Source: CAD feature listing. Evaluate the final solid. Frame: model axes, mm. A direction names the side the tool comes from. Round coordinates to 2 decimals unless told otherwise and drop trailing zeros. Loops run counter-clockwise (first coordinate to the right, second up) from the corner with the lowest first, then second, coordinate; pieces in that order, holes last. Notation, with made-up numbers: M 44,44 L 67,44 A8 cw 67,57 Z; hole C 44.25,-7 d7. An arc over 180 degrees is marked long. One line per item, written item: value.
from build123d import *

# Parameters (mm, degrees)
SKETCH_1_R      = 4
SKETCH_1_R_2    = 1.5
EXTRUDE_1_DEPTH = 3.3
SKETCH_2_W      = 33
SKETCH_2_H      = 26.5
SKETCH_2_R      = 4.9
SKETCH_2_R_2    = 1.495427909
EXTRUDE_2_DEPTH = 3.3


with BuildPart() as part:
    # 草图1 → 凸台-拉伸1 (new body)
    with BuildSketch(Plane(origin=(0, 0, 0), x_dir=(0, 0, -1), z_dir=(1, 0, 0))):
        with BuildLine():
            Line((-13.25, 0), (-13.25, -20.75))
            Line((-13.25, -20.75), (13.25, -20.75))
            Line((13.25, -20.75), (13.25, 0))
            ThreePointArc((13.25, 0), (0, 13.25), (-13.25, 0))
        make_face()
        Circle(SKETCH_1_R, mode=Mode.SUBTRACT)
        with Locations((8.5, 0)):
            Circle(SKETCH_1_R_2, mode=Mode.SUBTRACT)
        with Locations(Location((-8.5, 0, 0), (0, 0, 180))):
            Circle(SKETCH_1_R_2, mode=Mode.SUBTRACT)
    extrude(amount=EXTRUDE_1_DEPTH)

    # 草图2 → 凸台-拉伸2 (add)
    with BuildSketch(Plane.XZ.offset(20.75)):
        with Locations((16.5, 0)):
            Rectangle(SKETCH_2_W, SKETCH_2_H)
        with Locations(Location((17.8, 0, 0), (0, 0, 270))):
            Circle(SKETCH_2_R, mode=Mode.SUBTRACT)
        with Locations(Location((24.85, -8, 0), (0, 0, 270))):
            Circle(SKETCH_2_R_2, mode=Mode.SUBTRACT)
        with Locations(Location((24.85, 8, 0), (0, 0, 90))):
            Circle(SKETCH_2_R_2, mode=Mode.SUBTRACT)
        with Locations(Location((10.75, 8, 0), (0, 0, 270))):
            Circle(SKETCH_2_R_2, mode=Mode.SUBTRACT)
        with Locations(Location((10.75, -8, 0), (0, 0, 90))):
            Circle(SKETCH_2_R_2, mode=Mode.SUBTRACT)
    extrude(amount=-EXTRUDE_2_DEPTH)


solid = part.part
1. Section query A-A (x = 24.85). Return the cut outline in (y, z), and give its area (3 significant figures).
Report:
outline: M -20.75,-13.25 L -17.45,-13.25 L -17.45,-9.5 L -20.75,-9.5 Z; M -20.75,-6.5 L -17.45,-6.5 L -17.45,6.5 L -20.75,6.5 Z; M -20.75,9.5 L -17.45,9.5 L -17.45,13.25 L -20.75,13.25 Z
area: 67.7 mm2
2. Reachability of faces 1 (the face through (3.3, -5, 0)), 2 (the face through (12.6, -20.75, 0.2)) from +Z, -Z, +X, -X, +Y, -Y: full face, straight path, thin tool, end or side. Return the list, or none.
Report:
face 1: +Z, -Z, +X, +Y
face 2: +Z, -Z, +X, -X, -Y
3. Pull-direction query (Z, two-part tool) for faces 3 (the face through (18, -17.45, 6)), 4 (the face through (10, -18, 13.25)), 5 (the face through (1.6, -0.9, -7.3)), 6 (the face through (1.627, 13.247, -0.291)); classes: released by +Z, released by -Z, zero draft, split by the parting line, or undercut.
Report:
face 3: zero draft
face 4: released by +Z
face 5: undercut
face 6: split by the parting line
4. Ray query, line 1 (X direction, y = -19, z = -8); line 2 (X direction, y = -18.5, z = 0); line 3 (X direction, y = -14, z = 2). Return the intervals inside material, ascending. Write a range as [from, to].
Report:
line 1: x = [0, 9.25], [12.25, 23.35], [26.35, 33]
line 2: x = [0, 12.9], [22.7, 33]
line 3: x = [0, 3.3]
5. Pin query (flat end, axial travel): pin 1 (2.5 mm diameter, centred on x = 24.85, z = -8, fed in from -Y); pin 2 (3 mm diameter, centred on x = 16.5, z = 3.5, fed in from -Y); pin 3 (4 mm diameter, centred on x = 29, z = 7, fed in from +Y); pin 4 (3.5 mm diameter, centred on y = 0, z = 8.5, fed in from +X). Return the tip coordinate at first contact, or that it passes through.
Report:
pin 1: passes through
pin 2: stops at y = -20.75
pin 3: stops at y = -17.45
pin 4: stops at x = 3.3
6. Section query B-B (z = 0). Return the cut outline in (x, y).
Report:
outline: M 0,-20.75 L 12.9,-20.75 L 12.9,-17.45 L 3.3,-17.45 L 3.3,-4 L 0,-4 Z; M 0,4 L 3.3,4 L 3.3,13.25 L 0,13.25 Z; M 22.7,-20.75 L 33,-20.75 L 33,-17.45 L 22.7,-17.45 Z
7. Section query C-C (x = 17.8). Return the cut outline in (y, z).
Report:
outline: M -20.75,-13.25 L -17.45,-13.25 L -17.45,-4.9 L -20.75,-4.9 Z; M -20.75,4.9 L -17.45,4.9 L -17.45,13.25 L -20.75,13.25 Z
8. Section query D-D (z = -8). Return the cut outline in (x, y).
Report:
outline: M 0,-20.75 L 9.25,-20.75 L 9.25,-17.45 L 3.3,-17.45 L 3.3,-1.41 L 0,-1.41 Z; M 0,1.41 L 3.3,1.41 L 3.3,10.56 L 0,10.56 Z; M 12.25,-20.75 L 23.35,-20.75 L 23.35,-17.45 L 12.25,-17.45 Z; M 26.35,-20.75 L 33,-20.75 L 33,-17.45 L 26.35,-17.45 Z
